from build123d import *

# Parameters (mm, degrees)
F0_W          = 130
F0_H          = 70
F1_DEPTH      = 40
F2_W          = 124.4
F2_H          = 64.4
F3_DEPTH      = 38
F5_DEPTH      = 146.2
F6_W          = 130
F6_H          = 70
F6_W_2        = 127.2
F6_H_2        = 67.2
F7_DEPTH      = 10
F8_W          = 61
F8_H          = 46
F8_R          = 1.75
F9_DEPTH      = 25
F9_DEPTH_BACK = 25
F10_R         = 1.75
F11_DEPTH     = 25
F12_R         = 2.5
F12_R_2       = 1.75
F13_DEPTH     = 0.6
F14_R         = 1.2


with BuildPart() as f1:
    # F0 (on Top) → F1 (new body)
    with BuildSketch(Plane.XY):
        with Locations((-22.509574, 13.26069)):
            Rectangle(F0_W, F0_H)
    extrude(amount=F1_DEPTH)

    # F2 (on face) → F3 (cut)
    with BuildSketch(Plane.XY.offset(40)):
        with Locations((-22.509574, 13.26069)):
            Rectangle(F2_W, F2_H)
    extrude(amount=-F3_DEPTH, mode=Mode.SUBTRACT)

    # F4 (on face) → F5 (cut)
    with BuildSketch(Plane.YZ.offset(42.490426)):
        Polygon((48.26069, 40), (-11.73931, 40), (48.26069, 20), align=None)
    extrude(amount=-F5_DEPTH, mode=Mode.SUBTRACT)

    # F6 (on face) → F7 (cut)
    with BuildSketch(Plane(origin=(0, 0, 0), x_dir=(1, 0, 0), z_dir=(0, 0, -1))):
        with Locations((-22.509574, -13.26069)):
            Rectangle(F6_W, F6_H)
        with Locations((-22.509574, -13.26069)):
            Rectangle(F6_W_2, F6_H_2, mode=Mode.SUBTRACT)
    extrude(amount=-F7_DEPTH, mode=Mode.SUBTRACT)

    # F8 (on face) → F9 (cut, two sides)
    with BuildSketch(Plane.XY.offset(2)) as f9_sk:
        with Locations((-22.509574, 13.26069)):
            Rectangle(F8_W, F8_H)
        with Locations((-57.509574, 35.26069)):
            Circle(F8_R)
        with Locations((18.490426, 35.26069)):
            Circle(F8_R)
        with Locations((18.490426, -8.73931)):
            Circle(F8_R)
        with Locations((-57.509574, -8.73931)):
            Circle(F8_R)
    extrude(amount=-F9_DEPTH, mode=Mode.SUBTRACT)
    extrude(f9_sk.sketch, amount=-F9_DEPTH_BACK, mode=Mode.SUBTRACT)

    # F10 (on face) → F11 (cut)
    with BuildSketch(Plane.XY.offset(2)):
        with Locations((-80.709574, 41.46069)):
            Circle(F10_R)
        with Locations((35.690426, 41.46069)):
            Circle(F10_R)
        with Locations((35.690426, -14.93931)):
            Circle(F10_R)
        with Locations((-80.709574, -14.93931)):
            Circle(F10_R)
    extrude(amount=-F11_DEPTH, mode=Mode.SUBTRACT)

    # F12 (on face) → F13 (join)
    with BuildSketch(Plane.XY.offset(2)):
        with Locations((-57.509574, 35.26069)):
            Circle(F12_R)
        with Locations((-57.509574, 35.26069)):
            Circle(F12_R_2, mode=Mode.SUBTRACT)
        with Locations((18.490426, 35.26069)):
            Circle(F12_R)
        with Locations((18.490426, 35.26069)):
            Circle(F12_R_2, mode=Mode.SUBTRACT)
        with Locations((18.490426, -8.73931)):
            Circle(F12_R)
        with Locations((18.490426, -8.73931)):
            Circle(F12_R_2, mode=Mode.SUBTRACT)
        with Locations((-57.509574, -8.73931)):
            Circle(F12_R)
        with Locations((-57.509574, -8.73931)):
            Circle(F12_R_2, mode=Mode.SUBTRACT)
        with Locations((-80.709574, -14.93931)):
            Circle(F12_R)
        with Locations((-80.709574, -14.93931)):
            Circle(F12_R_2, mode=Mode.SUBTRACT)
        with Locations((-80.709574, 41.46069)):
            Circle(F12_R)
        with Locations((-80.709574, 41.46069)):
            Circle(F12_R_2, mode=Mode.SUBTRACT)
        with Locations((35.690426, 41.46069)):
            Circle(F12_R)
        with Locations((35.690426, 41.46069)):
            Circle(F12_R_2, mode=Mode.SUBTRACT)
        with Locations((35.690426, -14.93931)):
            Circle(F12_R)
        with Locations((35.690426, -14.93931)):
            Circle(F12_R_2, mode=Mode.SUBTRACT)
    extrude(amount=F13_DEPTH)

    # F14
    f14_edges = [f1.edges().sort_by_distance(p)[0] for p in [
        (39.690426, 45.46069, 11.466667),
        (-84.709574, 45.46069, 11.466667),
        (-84.709574, -18.93931, 21),
        (39.690426, -18.93931, 21),
        (-84.709574, 13.26069, 2),
        (-22.509574, -18.93931, 2),
        (39.690426, 13.26069, 2),
        (-22.509574, 45.46069, 2),
    ]]
    fillet(f14_edges, radius=F14_R)


solid = f1.part
Here's how the part is built. I have some questions about the finished solid (model axes, mm). A direction names the side the tool comes from. Coordinates: 2 decimals unless noted, no trailing zeros. Loops run counter-clockwise (first coordinate to the right, second up) from the corner with the lowest first, then second, coordinate; pieces in that order, holes last.
1. If we mould it in two halves opening along Y, with no side actions, what happens to faces 1 (the flat face through (-23, -21, 10)), 2 (the flat face through (-23, -21.739, 25)), 3 (the flat face through (39.69, 6, 18))? For each: pulls with the +Y half, pulls with the -Y half, needs draft (parallel to the pull), parting line crosses it, or undercut.
2. I need wall thicknesses on L1, parallel to X at y = 10, z = 30; L2, parallel to Y at x = -75.5, z = 16.5; L3, parallel to Y at x = -36, z = 5.5. Which ranges of each line are inside material? Lowest first, please.
3. Imagine slicing it at B-B, the plane y = 30. Please give me the cut outline in (x, z), and give its area (3 significant figures).
4. Imagine slicing it at A-A, the plane x = -50.5. Please give me the cut outline in (y, z), and give its area (3 significant figures).
5. Imagine slicing it at C-C, the plane x = -73. Please give me the cut outline in (y, z).
6. For faces 4 (the flat face through (-86.11, 14, 5)), 5 (the flat face through (-23, -20.339, 5)), 6 (the flat face through (42.49, 5, 21)), 7 (the flat face through (-22.206, 47.01, 20.417)), 8 (the cylindrical face through (38, 40.5, 2.3)), which set-ups out of +Z, -Z, +X, -X, +Y, -Y let a thin tool reach every point of the face, with its end or its side?
7. Imagine slicing it at D-D, the plane z = 35. Please give me the cut outline in (x, y), and give its area (3 significant figures).
8. For P1, Ø0.6, axis at x = -36.5, z = 0.5, coming from the +Y side; P2, Ø8, axis at x = -30, z = 7, coming from the +Y side; P3, Ø2, axis at x = -23.5, z = 1, coming from the -Y side; P4, Ø4, axis at x = -37.5, y = 39, coming from the +Z side, each with a flat end and sliding along its axis, tell me the tip position at first contact or that it passes through.
Taken from the geometry:
1. face 1: needs draft
1. face 2: pulls with the -Y half
1. face 3: undercut
2. L1: x = -87.51 to -84.71, 39.69 to 42.49
2. L2: y = -21.74 to -18.94, 45.46 to 48.26
2. L3: y = -20.34 to -18.94, 45.46 to 46.86
3. outline: (-87.51, 10) - (-86.11, 10) - (-86.11, 0) - (-53.01, 0) - (-53.01, 2) - (-83.51, 2) arc R1.2 cw to (-84.71, 3.2) - (-84.71, 26.09) - (-87.51, 26.09) - close; (7.99, 0) - (41.09, 0) - (41.09, 10) - (42.49, 10) - (42.49, 26.09) - (39.69, 26.09) - (39.69, 3.2) arc R1.2 cw to (38.49, 2) - (7.99, 2) - close
3. area: 246 mm2
4. outline: (-21.74, 10) - (-20.34, 10) - (-20.34, 0) - (-9.74, 0) - (-9.74, 2) - (-17.74, 2) arc R1.2 cw to (-18.94, 3.2) - (-18.94, 40) - (-21.74, 40) - close; (36.26, 0) - (46.86, 0) - (46.86, 10) - (48.26, 10) - (48.26, 20) - (45.46, 20.93) - (45.46, 3.2) arc R1.2 cw to (44.26, 2) - (36.26, 2) - close
4. area: 179 mm2
5. outline: (-21.74, 10) - (-20.34, 10) - (-20.34, 0) - (46.86, 0) - (46.86, 10) - (48.26, 10) - (48.26, 20) - (45.46, 20.93) - (45.46, 3.2) arc R1.2 cw to (44.26, 2) - (-17.74, 2) arc R1.2 cw to (-18.94, 3.2) - (-18.94, 40) - (-21.74, 40) - close
6. face 4: -Z, -X, +Y, -Y
6. face 5: -Z, +X, -X, -Y
6. face 6: +Z, -Z, +X, +Y, -Y
6. face 7: +Z, +X, -X, +Y
6. face 8: +Z
7. outline: (-87.51, -21.74) - (42.49, -21.74) - (42.49, 3.26) - (39.69, 3.26) - (39.69, -17.74) arc R1.2 cw to (38.49, -18.94) - (-83.51, -18.94) arc R1.2 cw to (-84.71, -17.74) - (-84.71, 3.26) - (-87.51, 3.26) - close
7. area: 489 mm2
8. P1: stops at y = 46.86
8. P2: stops at y = 48.26
8. P3: stops at y = -20.34
8. P4: stops at z = 2
